Source: three-view drawing plus pictorial views. Frame: mm from the lowest corner of the part. A direction names the side the tool comes from. Coordinates: 2 decimals unless noted, no trailing zeros. Loops run counter-clockwise (first coordinate to the right, second up) from the corner with the lowest first, then second, coordinate; pieces in that order, holes last.
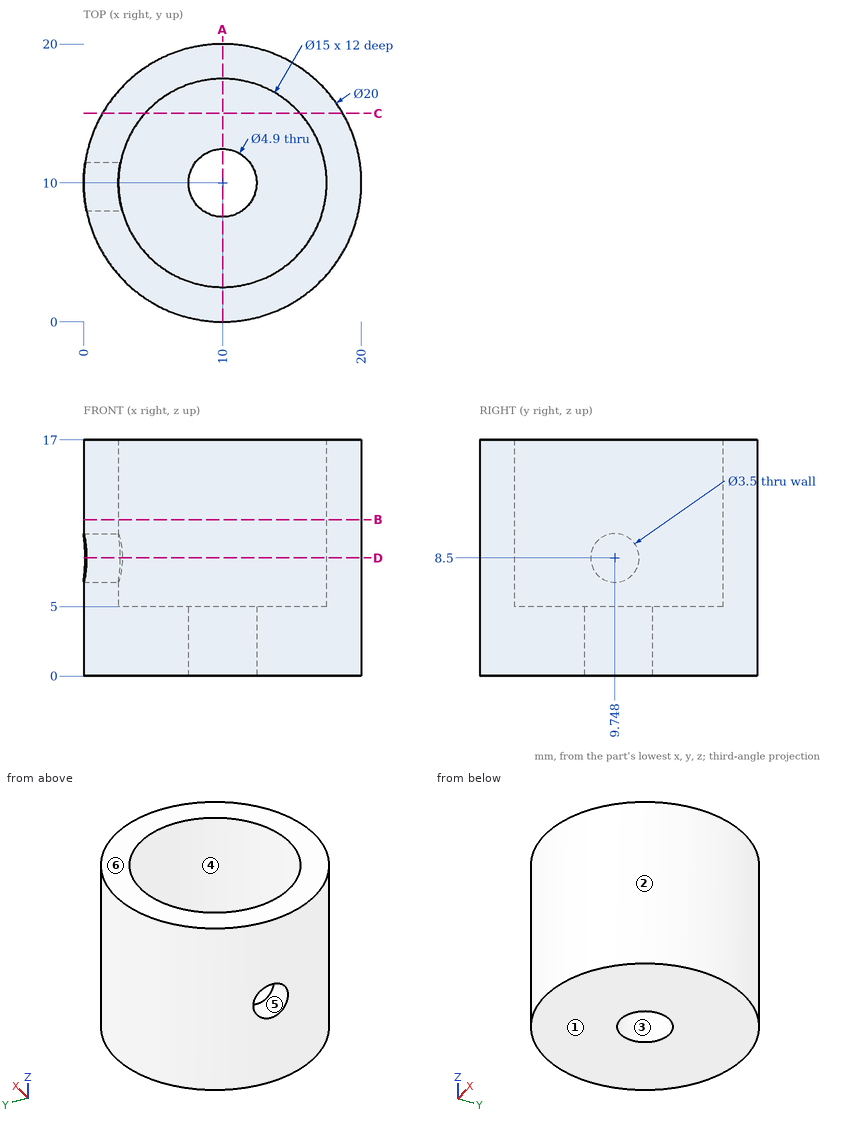
Q1. Material intervals for line 1 along Y through (x, z) = (10, 13.5); line 2 along Y through (x, z) = (10, 3.5); line 3 along Z through (x, y) = (5.5, 6.75), sorted ascending.
Q2. Section query B-B on z = 11.25. Return the cut outline in (x, y).
Q3. Section query C-C on y = 15. Return the cut outline in (x, z), then the cut area to 3 significant figures.
Q4. Section query A-A on x = 10. Return the cut outline in (y, z).
Q5. Section query D-D on z = 8.5. Return the cut outline in (x, y), then the cut area to 3 significant figures.
Q6. Reachability of the marked faces 4, 5 and 6 from +Z, -Z, +X, -X, +Y, -Y: full face, straight path, thin tool, end or side. Return the list, or none.
Q7. First-contact query: pin 1 Ø1 at (y, z) = (12, 14) entering from -X; pin 2 Ø10 at (y, z) = (17, 11) entering from +X; pin 3 Ø1.5 at (y, z) = (9, 4) entering from -X. Flat tips, straight axial feed; report the tip coordinate or a pass-through.
Q8. Draft query along X for the marked faces 1, 2 and 3. Return one class per face: released by +X, released by -X, zero draft, split by the parting line, or undercut.
Resolved:
1. line 1: y = 0 to 2.5, 17.5 to 20
1. line 2: y = 0 to 7.55, 12.45 to 20
1. line 3: z = 0 to 5
2. outline: circle Ø20 at (10, 10); hole circle Ø15 at (10, 10)
3. outline: (1.34, 0) - (18.66, 0) - (18.66, 17) - (15.59, 17) - (15.59, 5) - (4.41, 5) - (4.41, 17) - (1.34, 17) - close
3. area: 160 mm2
4. outline: (0, 0) - (7.55, 0) - (7.55, 5) - (2.5, 5) - (2.5, 17) - (0, 17) - close; (12.45, 0) - (20, 0) - (20, 17) - (17.5, 17) - (17.5, 5) - (12.45, 5) - close
5. outline: (0.11, 11.5) - (2.65, 11.5) arc R7.5 cw (long way) to (2.77, 8) - (0.2, 8) arc R10 ccw (long way) to start
5. area: 129 mm2
6. face 4: +Z
6. face 5: -X
6. face 6: +Z, +X, -X, +Y, -Y
7. pin 1: stops at x = 0.11
7. pin 2: stops at x = 19.8
7. pin 3: stops at x = 0
8. face 1: zero draft
8. face 2: split by the parting line
8. face 3: undercut
